Study the drawing (mm; zero at the part's minimum x, y, z) and answer. Give positions to 0.01 mm unless a question says otherwise; leave off trailing zeros. Loops run counter-clockwise (first coordinate to the right, second up) from the corner with the lowest first, then second, coordinate; pieces in that order, holes last. Notation, with made-up numbers: M -13,36 L -9,36 A16 cw -9,63 Z; hole C -1,74 d1. An arc over 180 degrees is marked long. Return JSON: item names as keys, results as strings.
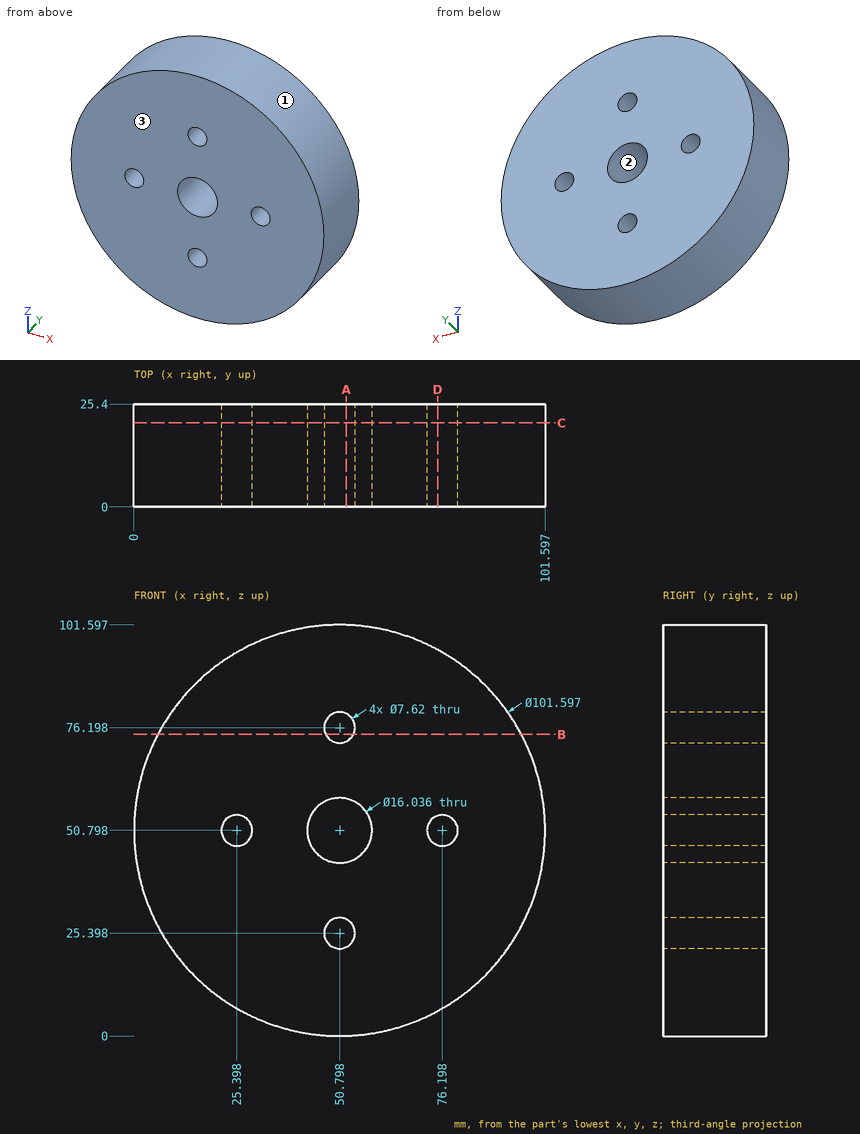
(1) Determine the mould class of the marked faces 1, 2 and 3 for opening direction X: released by +X, released by -X, zero draft, split by the parting line, or undercut.
Values follow:
{"face 1": "split by the parting line", "face 2": "undercut", "face 3": "zero draft"}
(2) The part is cut by section D-D (x = 75). Determine the outline of the cut face in (y, z) (1 decimal).
Values follow:
{"outline": "M 0,6.1 L 25.4,6.1 L 25.4,47.2 L 0,47.2 Z; M 0,54.4 L 25.4,54.4 L 25.4,95.5 L 0,95.5 Z"}
(3) The part is cut by section A-A (x = 52.5). Determine the outline of the cut face in (y, z).
Values follow:
{"outline": "M 0,0.03 L 25.4,0.03 L 25.4,21.99 L 0,21.99 Z; M 0,28.81 L 25.4,28.81 L 25.4,42.96 L 0,42.96 Z; M 0,58.63 L 25.4,58.63 L 25.4,72.79 L 0,72.79 Z; M 0,79.61 L 25.4,79.61 L 25.4,101.57 L 0,101.57 Z"}
(4) Given pin 1 (6 mm diameter, centred on y = 7, z = 84, fed in from -X); pin 2 (1.5 mm diameter, centred on y = 19.5, z = 69.5, fed in from +X); pin 3 (3 mm diameter, centred on y = 21, z = 51, fed in from -X); pin 4 (4 mm diameter, centred on x = 62.5, y = 19.5, fed in from -Z) (1 decimal), each flat-ended and moving along its own axis, determine where each tip first touches the part or whether it passes through.
Values follow:
{"pin 1": "x = 9.95", "pin 2": "x = 98.32", "pin 3": "x = 0", "pin 4": "z = 0.9"}
(5) The part is cut by section C-C (y = 20.75). Determine the outline of the cut face in (x, z).
Values follow:
{"outline": "C 50.8,50.8 d101.6; hole C 25.4,50.8 d7.62; hole C 50.8,50.8 d16.04; hole C 50.8,25.4 d7.62; hole C 50.8,76.2 d7.62; hole C 76.2,50.8 d7.62"}
(6) The part is cut by section B-B (z = 74.5). Determine the outline of the cut face in (x, y), and give its area (3 significant figures).
Values follow:
{"outline": "M 5.87,0 L 47.39,0 L 47.39,25.4 L 5.87,25.4 Z; M 54.21,0 L 95.73,0 L 95.73,25.4 L 54.21,25.4 Z", "area": "2,110 mm²"}
(7) Straight lines are drawn through the part: line 1 along Z through (x, y) = (58, 15.75) (1 decimal); line 2 along X through (y, z) = (18, 55.5) (1 decimal); line 3 along Z through (x, y) = (14.5, 15.5) (1 decimal). For each, find the intervals that lie inside material, in ascending order.
Values follow:
{"line 1": "0.5 to 47.3, 54.3 to 101.1", "line 2": "0.2 to 44.3, 57.3 to 101.4", "line 3": "15.3 to 86.3"}
